Read the model definition and answer for the solid it produces. Units are mm, in the model's axes. A direction names the side the tool comes from. Give positions to 0.01 mm unless a question says otherwise; leave off trailing zeros. Write each loop counter-clockwise with the first axis right and the second up, starting at its lowest first coordinate (ties: lowest second). Pieces come first, ordered by that corner, then holes. Notation, with made-up numbers: (75.25, 17.25) - (128.25, 17.25) arc R28 cw to (128.25, 39.25) - close; hole circle Ø4 at (36, 9). An arc over 180 degrees is marked (long way). Answer as a JSON object with one key per item and string values. Group by question number.
```python
from build123d import *

# Parameters (mm, degrees)
SKETCH_1_W          = 24
SKETCH_1_H          = 60
EXTRUDE_1_DEPTH     = 10
CHAMFER_1_SIZE      = 2
SKETCH_3_R          = 2.1
CUT_EXTRUDE_1_DEPTH = 15
SKETCH_4_R          = 5
CUT_EXTRUDE_2_DEPTH = 6


with BuildPart() as part:
    # 草图1 → 凸台-拉伸1 (new body)
    with BuildSketch(Plane(origin=(0, 0, 0), x_dir=(1, 0, 0), z_dir=(0, 1, 0))):
        Rectangle(SKETCH_1_W, SKETCH_1_H)
    extrude(amount=EXTRUDE_1_DEPTH)

    # 倒角1
    chamfer_1_edges = [part.edges().sort_by_distance(p)[0] for p in [
        (12, 5, 30),
        (-12, 5, 30),
        (-12, 5, -30),
        (12, 5, -30),
    ]]
    chamfer(chamfer_1_edges, length=CHAMFER_1_SIZE)

    # 草图3 → 切除-拉伸1 (cut)
    with BuildSketch(Plane(origin=(0, 10, 0), x_dir=(1, 0, 0), z_dir=(0, 1, 0))):
        with Locations(Location((0, -8, 0), (0, 0, 270))):
            Circle(SKETCH_3_R)
        with Locations(Location((0, 8, 0), (0, 0, 270))):
            Circle(SKETCH_3_R)
        with Locations(Location((0, -24, 0), (0, 0, 270))):
            Circle(SKETCH_3_R)
        with Locations(Location((0, 24, 0), (0, 0, 270))):
            Circle(SKETCH_3_R)
    extrude(amount=-CUT_EXTRUDE_1_DEPTH, mode=Mode.SUBTRACT)

    # 草图4 → 切除-拉伸2 (cut)
    with BuildSketch(Plane.XZ):
        with Locations(Location((0, -24, 0), (0, 0, 270))):
            Circle(SKETCH_4_R)
        with Locations(Location((0, -8, 0), (0, 0, 270))):
            Circle(SKETCH_4_R)
        with Locations(Location((0, 8, 0), (0, 0, 270))):
            Circle(SKETCH_4_R)
        with Locations(Location((0, 24, 0), (0, 0, 270))):
            Circle(SKETCH_4_R)
    extrude(amount=-CUT_EXTRUDE_2_DEPTH, mode=Mode.SUBTRACT)


solid = part.part
```
1) Which of the six approach directions +Z, -Z, +X, -X, +Y, -Y give full straight-line access (tool end or side, diameter ignored) to faces 1 (the flat face through (11, 5, -29)), 2 (the cylindrical face through (1.5, 2.96, 3.23))?
2) Find section C-C, the plane z = -24. Write down the section's boundary in (x, y).
3) For a pull along Z with two mould halves and no side action, classify faces 3 (the flat face through (0, 5, -30)), 4 (the cylindrical face through (-0.8, 8.03, 25.94)), 5 (the flat face through (11, 5, 29)), 6 (the cylindrical face through (0.09, 8.03, 5.9)) as released by +Z, released by -Z, zero draft, split by the parting line, or undercut.
4) Flat-ended cylindrical pins translate along their axes: pin 1 Ø5 at (x, z) = (-0.5, 5.5) entering from -Y; pin 2 Ø5 at (x, z) = (1.5, -23) entering from -Y. Find the tip coordinate at first contact, or state that the pin passes through.
5) Find section D-D, the plane y = 6.75. Write down the section's boundary in (x, z), and give its area (3 significant figures).
6) Find section A-A, the plane y = 2. Write down the section's boundary in (x, z), and give its area (3 significant figures).
7) Find section B-B, the plane x = 3. Write down the section's boundary in (y, z), and give its area (3 significant figures).
8) Find the intervals of material crossed by line 1 (X direction, y = 2.55, z = -24); line 2 (X direction, y = 8.7, z = 8); line 3 (Z direction, x = -0.25, y = 8.25), in increasing order. Write a range as [from, to].
Values follow:
{
 "1": {"face 1": "-Z, +X, +Y, -Y", "face 2": "-Y"},
 "2": {"outline": "(-12, 0) - (-5, 0) - (-5, 6) - (-2.1, 6) - (-2.1, 10) - (-12, 10) - close; (2.1, 6) - (5, 6) - (5, 0) - (12, 0) - (12, 10) - (2.1, 10) - close"},
 "3": {"face 3": "released by -Z", "face 4": "undercut", "face 5": "released by +Z", "face 6": "undercut"},
 "4": {"pin 1": "stops at y = 0", "pin 2": "stops at y = 6"},
 "5": {"outline": "(-12, -28) - (-10, -30) - (10, -30) - (12, -28) - (12, 28) - (10, 30) - (-10, 30) - (-12, 28) - close; hole circle Ø4.2 at (0, -24); hole circle Ø4.2 at (0, -8); hole circle Ø4.2 at (0, 8); hole circle Ø4.2 at (0, 24)", "area": "1,380 mm2"},
 "6": {"outline": "(-12, -28) - (-10, -30) - (10, -30) - (12, -28) - (12, 28) - (10, 30) - (-10, 30) - (-12, 28) - close; hole circle Ø10 at (0, -24); hole circle Ø10 at (0, -8); hole circle Ø10 at (0, 8); hole circle Ø10 at (0, 24)", "area": "1,120 mm2"},
 "7": {"outline": "(0, -30) - (10, -30) - (10, 30) - (0, 30) - (0, 28) - (6, 28) - (6, 20) - (0, 20) - (0, 12) - (6, 12) - (6, 4) - (0, 4) - (0, -4) - (6, -4) - (6, -12) - (0, -12) - (0, -20) - (6, -20) - (6, -28) - (0, -28) - close", "area": "408 mm2"},
 "8": {"line 1": "x = [-12, -5], [5, 12]", "line 2": "x = [-12, -2.1], [2.1, 12]", "line 3": "z = [-30, -26.09], [-21.91, -10.09], [-5.91, 5.91], [10.09, 21.91], [26.09, 30]"}
}
